Build history of the part. All positions in model axes, mm. A direction names the side the tool comes from. Give positions to 0.01 mm unless a question says otherwise; leave off trailing zeros. Order: outer loops, then holes, each group sorted by start corner. A loop starts at its lowest first (then second) coordinate and runs counter-clockwise, first axis right, second up. Notation, with made-up numbers: (46, 67.5) - (73, 67.5) arc R19 cw to (73, 77.5) - close; hole circle Ø9 at (77.5, 26.5). An arc over 180 degrees is marked (long way). Use a Markdown table: item, result. Add a question column.
(1) Slice it at B-B (z = 4.25). Count the separate pieces of the cut face and the enclosed holes in it, then the cut area to 3 significant figures.
(2) Mould opens along X. For faces 3 (the face through (-1, 3, 0)), 4 (the face through (35.47, -3.93, 4.93)) say: +X half, -X half, draft (parallel to the pull), parting line (faces both ways), or undercut.
(3) Slice it at A-A (x = 1). Write the cut outline in (y, z), then the cut area to 3 significant figures.
(4) Flat gauge pins, fed straight in: pin 1 (3 mm diameter, centred on x = 30, z = 3.5, fed in from +Y); pin 2 (2 mm diameter, centred on x = -6, z = 2.5, fed in from +Y); pin 3 (6 mm diameter, centred on x = 22, z = 4.5, fed in from -Y). Where does each tip first touch, or does it go through?
(5) Wall check: line 1 (Y direction, x = 0, z = 7.25); line 2 (X direction, y = -4.5, z = 1.25); line 3 (X direction, y = -1, z = 0.75) (3 decimals). Give the ranges that are in metal, low to high.
(6) Slice it at D-D (y = 36.5). Write the cut outline in (x, z).
(7) Slice it at C-C (x = -21.5). Write the cut outline in (y, z), then the cut area to 3 significant figures.
(8) Which spindle directions (+Z, -Z, +X, -X, +Y, -Y) get a long thin tool onto all of the face, cutting with end or side? Do faces 1 (the face through (-1, 3, 10)), 2 (the face through (31, -7.909, 5)). Say none if no direction does.
from build123d import *

# Parameters (mm, degrees)
F1_DEPTH = 10


with BuildPart() as f1:
    # F0 (on Top) → F1 (new body)
    with BuildSketch(Plane.XY):
        with BuildLine():
            ThreePointArc((40.4156393511, -7.9090867682), (41.3673030509, -2.8418043205), (41.6861501393, 2.3041991517))
            ThreePointArc((41.6861501393, 2.3041991517), (-5.1460034722, 43.6715022026), (-40.4156393511, -7.9090867682))
            Line((-40.4156393511, -7.9090867682), (-40.4156393511, 0))
            Line((-40.4156393511, 0), (-37.1771354638, 0))
            add(Edge.make_bspline(
                [(-37.1771354638, 0), (-36.8978650572, 0.0446259236), (-36.5915409745, 0.0446259236)],
                knots=[0.6161917381, 0.6161917381, 0.6161917381, 1, 1, 1], degree=2))
            add(Edge.make_bspline(
                [(-36.5915409745, 0.0446259236), (-36.2539809593, 0.0446259236), (-35.9330292975, 0)],
                knots=[0, 0, 0, 0.2900730853, 0.2900730853, 0.2900730853], degree=2))
            Line((-35.9330292975, 0), (17.3402957465, 0))
            add(Edge.make_bspline(
                [(17.3402957465, 0), (17.6195661531, 0.0446259236), (17.9258902358, 0.0446259236)],
                knots=[0.6161917381, 0.6161917381, 0.6161917381, 1, 1, 1], degree=2))
            add(Edge.make_bspline(
                [(17.9258902358, 0.0446259236), (18.263450251, 0.0446259236), (18.5844019128, 0)],
                knots=[0, 0, 0, 0.2900730853, 0.2900730853, 0.2900730853], degree=2))
            Line((18.5844019128, 0), (24.0306765024, 0))
            add(Edge.make_bspline(
                [(24.0306765024, 0), (24.369078423, 0.0566405953), (24.7330599673, 0.0566405953)],
                knots=[0.7021583014, 0.7021583014, 0.7021583014, 1, 1, 1], degree=2))
            add(Edge.make_bspline(
                [(24.7330599673, 0.0566405953), (25.1035042565, 0.0566405953), (25.4286990035, 0)],
                knots=[0, 0, 0, 0.2708012802, 0.2708012802, 0.2708012802], degree=2))
            Line((25.4286990035, 0), (40.4156393511, 0))
            Line((40.4156393511, 0), (40.4156393511, -7.9090867682))
        make_face()
        with BuildLine():
            Line((-39.3036225538, -7.9090867682), (-40.4156393511, -7.9090867682))
            ThreePointArc((-40.4156393511, -7.9090867682), (0, -39.3819509876), (40.4156393511, -7.9090867682))
            Line((40.4156393511, -7.9090867682), (37.7818098534, -7.9090867682))
            add(Edge.make_bspline(
                [(37.7818098534, -7.9090867682), (37.5360380286, -8.053262829), (37.1991400882, -8.053262829)],
                knots=[0.2939431181, 0.2939431181, 0.2939431181, 1, 1, 1], degree=2))
            add(Edge.make_bspline(
                [(37.1991400882, -8.053262829), (36.8661003441, -8.053262829), (36.6575202765, -7.9090867682)],
                knots=[0, 0, 0, 0.8473185457, 0.8473185457, 0.8473185457], degree=2))
            Line((36.6575202765, -7.9090867682), (34.6297167175, -7.9090867682))
            Line((34.6297167175, -7.9090867682), (32.7949047047, -7.9090867682))
            Line((32.7949047047, -7.9090867682), (29.7002685409, -7.9090867682))
            Line((29.7002685409, -7.9090867682), (28.2258966802, -7.9090867682))
            Line((28.2258966802, -7.9090867682), (24.4546855592, -7.9090867682))
            add(Edge.make_bspline(
                [(24.4546855592, -7.9090867682), (23.9989033781, -8.0172188138), (23.4938323964, -8.0172188138)],
                knots=[0.5796214889, 0.5796214889, 0.5796214889, 1, 1, 1], degree=2))
            add(Edge.make_bspline(
                [(23.4938323964, -8.0172188138), (22.9862299942, -8.0172188138), (22.5610753448, -7.9090867682)],
                knots=[0, 0, 0, 0.3696747706, 0.3696747706, 0.3696747706], degree=2))
            Line((22.5610753448, -7.9090867682), (17.2428330681, -7.9090867682))
            add(Edge.make_bspline(
                [(17.2428330681, -7.9090867682), (16.7839236692, -8.0172188138), (16.2318215205, -8.0172188138)],
                knots=[0.5928274645, 0.5928274645, 0.5928274645, 1, 1, 1], degree=2))
            add(Edge.make_bspline(
                [(16.2318215205, -8.0172188138), (15.671241471, -8.0172188138), (15.2138086565, -7.9090867682)],
                knots=[0, 0, 0, 0.4726565934, 0.4726565934, 0.4726565934], degree=2))
            Line((15.2138086565, -7.9090867682), (12.4883930827, -7.9090867682))
            Line((12.4883930827, -7.9090867682), (10.8526813444, -7.9090867682))
            Line((10.8526813444, -7.9090867682), (5.8374140839, -7.9090867682))
            Line((5.8374140839, -7.9090867682), (3.4190323008, -7.9090867682))
            Line((3.4190323008, -7.9090867682), (-1.5962349597, -7.9090867682))
            Line((-1.5962349597, -7.9090867682), (-4.0146167428, -7.9090867682))
            Line((-4.0146167428, -7.9090867682), (-4.9603430469, -7.9090867682))
            Line((-4.9603430469, -7.9090867682), (-6.5531452432, -7.9090867682))
            Line((-6.5531452432, -7.9090867682), (-10.1403829484, -7.9090867682))
            Line((-10.1403829484, -7.9090867682), (-11.8567646255, -7.9090867682))
            Line((-11.8567646255, -7.9090867682), (-14.7128237363, -7.9090867682))
            Line((-14.7128237363, -7.9090867682), (-16.3056259326, -7.9090867682))
            Line((-16.3056259326, -7.9090867682), (-19.8928636378, -7.9090867682))
            Line((-19.8928636378, -7.9090867682), (-21.6092453149, -7.9090867682))
            Line((-21.6092453149, -7.9090867682), (-22.2374410087, -7.9090867682))
            Line((-22.2374410087, -7.9090867682), (-26.6193634304, -7.9090867682))
            Line((-26.6193634304, -7.9090867682), (-28.5073832753, -7.9090867682))
            Line((-28.5073832753, -7.9090867682), (-30.1482441586, -7.9090867682))
            Line((-30.1482441586, -7.9090867682), (-32.6747579873, -7.9090867682))
            Line((-32.6747579873, -7.9090867682), (-34.3104697256, -7.9090867682))
            Line((-34.3104697256, -7.9090867682), (-37.2745981422, -7.9090867682))
            add(Edge.make_bspline(
                [(-37.2745981422, -7.9090867682), (-37.7335075411, -8.0172188138), (-38.2856096898, -8.0172188138)],
                knots=[0.5928274645, 0.5928274645, 0.5928274645, 1, 1, 1], degree=2))
            add(Edge.make_bspline(
                [(-38.2856096898, -8.0172188138), (-38.8461897393, -8.0172188138), (-39.3036225538, -7.9090867682)],
                knots=[0, 0, 0, 0.4726565934, 0.4726565934, 0.4726565934], degree=2))
        make_face()
        with BuildLine():
            Line((-40.4156393511, 0), (-40.4156393511, -7.9090867682))
            Line((-40.4156393511, -7.9090867682), (-39.3036225538, -7.9090867682))
            add(Edge.make_bspline(
                [(-39.3036225538, -7.9090867682), (-39.8139807759, -7.788443743), (-40.1959424964, -7.5331991809)],
                knots=[0.4726565934, 0.4726565934, 0.4726565934, 1, 1, 1], degree=2))
            Line((-40.1959424964, -7.5331991809), (-40.1959424964, -6.0639764653))
            add(Edge.make_bspline(
                [(-40.1959424964, -6.0639764653), (-39.1609643451, -6.6423970904), (-38.2753113997, -6.6423970904)],
                knots=[0, 0, 0, 1, 1, 1], degree=2))
            add(Edge.make_bspline(
                [(-38.2753113997, -6.6423970904), (-37.6745778127, -6.6423970904), (-37.3364506223, -6.4149765182)],
                knots=[0, 0, 0, 1, 1, 1], degree=2))
            add(Edge.make_bspline(
                [(-37.3364506223, -6.4149765182), (-36.998323432, -6.187555946), (-36.998323432, -5.7910717786)],
                knots=[0, 0, 0, 1, 1, 1], degree=2))
            add(Edge.make_bspline(
                [(-36.998323432, -5.7910717786), (-36.998323432, -5.5593602522), (-37.0712696532, -5.385147512)],
                knots=[0, 0, 0, 1, 1, 1], degree=2))
            add(Edge.make_bspline(
                [(-37.0712696532, -5.385147512), (-37.1442158745, -5.2109347717), (-37.2780936453, -5.060751375)],
                knots=[0, 0, 0, 1, 1, 1], degree=2))
            add(Edge.make_bspline(
                [(-37.2780936453, -5.060751375), (-37.4119714161, -4.9105679782), (-37.9423333544, -4.5140838108)],
                knots=[0, 0, 0, 1, 1, 1], degree=2))
            add(Edge.make_bspline(
                [(-37.9423333544, -4.5140838108), (-38.6838102389, -3.9820054909), (-38.9841770324, -3.4619418427)],
                knots=[0, 0, 0, 1, 1, 1], degree=2))
            add(Edge.make_bspline(
                [(-38.9841770324, -3.4619418427), (-39.2845438259, -2.9418781946), (-39.2845438259, -2.3411446076)],
                knots=[0, 0, 0, 1, 1, 1], degree=2))
            add(Edge.make_bspline(
                [(-39.2845438259, -2.3411446076), (-39.2845438259, -1.6494427917), (-38.9515657805, -1.1053498001)],
                knots=[0, 0, 0, 1, 1, 1], degree=2))
            add(Edge.make_bspline(
                [(-38.9515657805, -1.1053498001), (-38.6185877352, -0.5612568084), (-38.0041230947, -0.2583154424)],
                knots=[0, 0, 0, 1, 1, 1], degree=2))
            add(Edge.make_bspline(
                [(-38.0041230947, -0.2583154424), (-37.6254950599, -0.0716454755), (-37.1771354638, 0)],
                knots=[0, 0, 0, 0.6161917381, 0.6161917381, 0.6161917381], degree=2))
            Line((-37.1771354638, 0), (-40.4156393511, 0))
        make_face()
        with BuildLine():
            Line((37.7818098534, -7.9090867682), (40.4156393511, -7.9090867682))
            Line((40.4156393511, -7.9090867682), (40.4156393511, 0))
            Line((40.4156393511, 0), (25.4286990035, 0))
            add(Edge.make_bspline(
                [(25.4286990035, 0), (26.3043654444, -0.1525186646), (26.8519331477, -0.7157311594)],
                knots=[0.2708012802, 0.2708012802, 0.2708012802, 1, 1, 1], degree=2))
            add(Edge.make_bspline(
                [(26.8519331477, -0.7157311594), (27.6028501314, -1.4881029141), (27.6028501314, -2.8783720725)],
                knots=[0, 0, 0, 1, 1, 1], degree=2))
            add(Edge.make_bspline(
                [(27.6028501314, -2.8783720725), (27.6028501314, -4.3956534751), (27.0716300023, -5.5945460766)],
                knots=[0, 0, 0, 1, 1, 1], degree=2))
            add(Edge.make_bspline(
                [(27.0716300023, -5.5945460766), (26.5404098733, -6.793438678), (25.6178547218, -7.4053287459)],
                knots=[0, 0, 0, 1, 1, 1], degree=2))
            add(Edge.make_bspline(
                [(25.6178547218, -7.4053287459), (25.0831219313, -7.7599933781), (24.4546855592, -7.9090867682)],
                knots=[0, 0, 0, 0.5796214889, 0.5796214889, 0.5796214889], degree=2))
            Line((24.4546855592, -7.9090867682), (28.2258966802, -7.9090867682))
            Line((28.2258966802, -7.9090867682), (29.8822049986, -0.0669388854))
            Line((29.8822049986, -0.0669388854), (31.7976869503, -0.0669388854))
            Line((31.7976869503, -0.0669388854), (33.6204842914, -5.8442796106))
            Line((33.6204842914, -5.8442796106), (33.6427972532, -5.8442796106))
            add(Edge.make_bspline(
                [(33.6427972532, -5.8442796106), (33.7063033752, -5.4357807714), (33.851337627, -4.6797146427)],
                knots=[0, 0, 0, 1, 1, 1], degree=2))
            add(Edge.make_bspline(
                [(33.851337627, -4.6797146427), (33.9963718787, -3.9236485139), (34.8168023203, -0.0669388854)],
                knots=[0, 0, 0, 1, 1, 1], degree=2))
            Line((34.8168023203, -0.0669388854), (36.2877414176, -0.0669388854))
            Line((36.2877414176, -0.0669388854), (34.6297167175, -7.9090867682))
            Line((34.6297167175, -7.9090867682), (36.6575202765, -7.9090867682))
            add(Edge.make_bspline(
                [(36.6575202765, -7.9090867682), (36.6199354647, -7.8831071519), (36.5863918294, -7.8524461728)],
                knots=[0.8473185457, 0.8473185457, 0.8473185457, 1, 1, 1], degree=2))
            add(Edge.make_bspline(
                [(36.5863918294, -7.8524461728), (36.3666949748, -7.6516295166), (36.3666949748, -7.2929057461)],
                knots=[0, 0, 0, 1, 1, 1], degree=2))
            add(Edge.make_bspline(
                [(36.3666949748, -7.2929057461), (36.3666949748, -6.8088861131), (36.6541889057, -6.5196758005)],
                knots=[0, 0, 0, 1, 1, 1], degree=2))
            add(Edge.make_bspline(
                [(36.6541889057, -6.5196758005), (36.9416828366, -6.2304654879), (37.4617464848, -6.2304654879)],
                knots=[0, 0, 0, 1, 1, 1], degree=2))
            add(Edge.make_bspline(
                [(37.4617464848, -6.2304654879), (37.8256194003, -6.2304654879), (38.045316255, -6.4338567167)],
                knots=[0, 0, 0, 1, 1, 1], degree=2))
            add(Edge.make_bspline(
                [(38.045316255, -6.4338567167), (38.2650131097, -6.6372479454), (38.2650131097, -7.0079863877)],
                knots=[0, 0, 0, 1, 1, 1], degree=2))
            add(Edge.make_bspline(
                [(38.2650131097, -7.0079863877), (38.2650131097, -7.4748422038), (37.970653652, -7.7640525164)],
                knots=[0, 0, 0, 1, 1, 1], degree=2))
            add(Edge.make_bspline(
                [(37.970653652, -7.7640525164), (37.8841287152, -7.8490638975), (37.7818098534, -7.9090867682)],
                knots=[0, 0, 0, 0.2939431181, 0.2939431181, 0.2939431181], degree=2))
        make_face()
        Polygon((39.7033409551, -0.0669388854), (38.3302356134, -5.3070521456), (37.0378002105, -5.3070521456), (37.8788272323, -0.0669388854), align=None, mode=Mode.SUBTRACT)
    extrude(amount=F1_DEPTH)


solid = f1.part
Solution:
| question | item | result |
|---|---|---|
| 1 | separate pieces | 1 |
| 1 | enclosed holes | 4 |
| 1 | area | 4,890 mm2 |
| 2 | face 3 | draft |
| 2 | face 4 | undercut |
| 3 | outline | (-39.37, 0) - (-7.91, 0) - (-7.91, 10) - (-39.37, 10) - close; (0, 0) - (43.98, 0) - (43.98, 10) - (0, 10) - close |
| 3 | area | 754 mm2 |
| 4 | pin 1 | y = 32.73 |
| 4 | pin 2 | y = 43.69 |
| 4 | pin 3 | y = -34.8 |
| 5 | line 1 | -39.38 to -7.91, 0 to 43.99 |
| 5 | line 2 | -41.13 to -37.96, 27.43 to 28.95, 33.2 to 33.89, 35.35 to 37.17, 38.54 to 41.13 |
| 5 | line 3 | -41.555 to -38.883, 27.088 to 29.685, 32.092 to 34.619, 36.09 to 37.729, 39.459 to 41.555 |
| 6 | outline | (-23.84, 0) - (23.84, 0) - (23.84, 10) - (-23.84, 10) - close |
| 7 | outline | (-33.41, 0) - (-7.91, 0) - (-7.91, 10) - (-33.41, 10) - close; (0, 0) - (38.02, 0) - (38.02, 10) - (0, 10) - close |
| 7 | area | 635 mm2 |
| 8 | face 1 | +Z, +X, -X, +Y, -Y |
| 8 | face 2 | +Z, -Z |
